Part model, mm, in its own coordinate system. Round coordinates to 2 decimals unless told otherwise and drop trailing zeros. Order: outer loops, then holes, each group sorted by start corner. A loop starts at its lowest first (then second) coordinate and runs counter-clockwise, first axis right, second up. Notation, with made-up numbers: (25.25, -29) - (66.25, -29) arc R8 cw to (66.25, -24) - close; hole circle Ø3 at (27.5, -9.75). An arc over 180 degrees is marked (long way). Return JSON: item names as keys, results as strings. Group by question number.
Item 1: Probe probe 1 along Y at (x, z) = (84.9, 0.75); probe 2 along X at (y, z) = (-13, 0.55); probe 3 along X at (y, z) = (-20.25, 1.1). List the from-to ranges inside material, lowest first.
Item 2: Two-plate mould, pull along X, no slides. Class faces 1 (the face through (34.4, -10.7, 1.4)), 2 (the face through (82.8, -19.71, 0.44)), 3 (the face through (0.45, -0.43, 0.69)): released by +X, released by -X, zero draft, split by the parting line, or undercut.
Item 3: Saw through at B-B on z = 0.45. List the corners of the cut face in (x, y).
Item 4: Saw through at A-A on x = 84.9. List the corners of the cut face in (y, z).
Item 5: Saw through at C-C on x = 59. List the corners of the cut face in (y, z), and give its area (3 significant figures).
Item 6: Drop a flat-ended pin along its axis: pin 1 (10 mm diameter, centred on x = 47.5, y = -19, fed in from +Z) (1 decimal). Give the stop position or say it passes through.
```python
from build123d import *

# Parameters (mm, degrees)
F0_R     = 2.1
F1_DEPTH = 1.4
F2_SIZE  = 0.5


with BuildPart() as f1:
    # F0 (on Top) → F1 (new body)
    with BuildSketch(Plane.XY):
        with BuildLine():
            Line((88.5, 0), (1.5, 0))
            ThreePointArc((1.5, 0), (0.43934, -0.43934), (0, -1.5))
            Line((0, -1.5), (0, -28))
            Line((0, -28), (33, -28))
            Line((33, -28), (33, -11))
            Line((33, -11), (81.25, -11))
            Line((81.25, -11), (81.25, -28))
            Line((81.25, -28), (90, -28))
            Line((90, -28), (90, -1.5))
            ThreePointArc((90, -1.5), (89.56066, -0.43934), (88.5, 0))
        make_face()
        with Locations((29.93, -19.6)):
            Circle(F0_R, mode=Mode.SUBTRACT)
        with Locations((84.9, -19.8)):
            Circle(F0_R, mode=Mode.SUBTRACT)
    extrude(amount=F1_DEPTH)

    # F2
    f2_edges = [f1.edges().sort_by_distance(p)[0] for p in [
        (27.83, -19.6, 1.4),
        (82.8, -19.8, 1.4),
    ]]
    chamfer(f2_edges, length=F2_SIZE)


solid = f1.part
```
Filled in:
{
 "1": {"probe 1": "y = -28 to -21.9, -17.7 to 0", "probe 2": "x = 0 to 33, 81.25 to 90", "probe 3": "x = 0 to 27.72, 32.14 to 33, 81.25 to 82.64, 87.16 to 90"},
 "2": {"face 1": "zero draft", "face 2": "undercut", "face 3": "released by -X"},
 "3": {"outline": "(0, -28) - (33, -28) - (33, -11) - (81.25, -11) - (81.25, -28) - (90, -28) - (90, -1.5) arc R1.5 ccw to (88.5, 0) - (1.5, 0) arc R1.5 ccw to (0, -1.5) - close; hole circle Ø4.2 at (29.93, -19.6); hole circle Ø4.2 at (84.9, -19.8)"},
 "4": {"outline": "(-28, 0) - (-21.9, 0) - (-21.9, 0.9) - (-22.4, 1.4) - (-28, 1.4) - close; (-17.7, 0) - (0, 0) - (0, 1.4) - (-17.2, 1.4) - (-17.7, 0.9) - close"},
 "5": {"outline": "(-11, 0) - (0, 0) - (0, 1.4) - (-11, 1.4) - close", "area": "15.4 mm^2"},
 "6": {"pin 1": "passes through"}
}
